Input: part model. Units: mm. Frame: model coordinates. Face numbers are marked on the shaded views. A direction names the side the tool comes from. Round coordinates to 2 decimals unless told otherwise and drop trailing zeros. Loops run counter-clockwise (first coordinate to the right, second up) from the corner with the lowest first, then second, coordinate; pieces in that order, holes last. Notation, with made-up numbers: (76, -35) -> (91, -35) arc R27 cw to (91, -4) -> close; hole circle Ø5 at (-21.5, -36.5). An arc over 180 degrees is marked (long way). Answer in a Markdown table with one row per item. Add a question column.
Q1. Pin query (flat end, axial travel): pin 1 (6 mm diameter, centred on y = -5.5, z = 9.5, fed in from +X); pin 2 (5 mm diameter, centred on x = 10.5, z = 38, fed in from -Y); pin 3 (5 mm diameter, centred on x = 11, z = 13.5, fed in from +Y). Return the tip coordinate at first contact, or that it passes through.
Q2. Section B-B, the plane y = -13.5. Output: boundary loops of the cut face in (x, z), and give its area (3 significant figures).
Q3. Ray query, L1, parallel to Y at x = 20.75, z = 8.5 (3 decimals); L2, parallel to X at y = -14.75, z = 41.5; L3, parallel to Z at x = 18.5, y = -10.5. Return the intervals inside material, ascending. Write a range as from..to.
Q4. Section A-A, the plane z = 11.5. Output: boundary loops of the cut face in (x, y) (3 decimals), and give its area (3 significant figures).
Q5. Reachability of the marked faces 1, 2 and 3 from +Z, -Z, +X, -X, +Y, -Y: full face, straight path, thin tool, end or side. Return the list, or none.
Q6. Mould query, pull axis X, two halves, no side actions, for the marked faces 4, 5, 6 and 7. Classes: pulls with the +X half, pulls with the -X half, needs draft (parallel to the pull), parting line crosses it, or undercut.
Q7. Section C-C, the plane x = 20.25. Output: boundary loops of the cut face in (y, z) (3 decimals).
Q8. Section D-D, the plane z = 7. Output: boundary loops of the cut face in (x, y).
```python
from build123d import *

# Parameters (mm, degrees)
F0_W      = 25.4
F0_H      = 25.4
F1_DEPTH  = 5.08
F2_W      = 20.32
F2_H      = 20.32
F3_DEPTH  = 2.54
F4_W      = 10.16
F4_H      = 10.16
F5_DEPTH  = 10.16
F6_W      = 5.08
F6_H      = 5.08
F7_DEPTH  = 25.4
F8_W      = 2.54
F8_H      = 2.54
F9_DEPTH  = 5.08
F10_R     = 0.635
F11_DEPTH = 0.254
F13_R     = 2.2046300475
F14_DEPTH = 25.4


# Not quite as in the source:
# - a fillet or chamfer that OpenCascade refuses, or shapes differently, is made with other operations: its cross-section is extruded or revolved along the edge and cut away or added


with BuildPart() as f1:
    # F0 (on Top) → F1 (new body)
    with BuildSketch(Plane.XY):
        with Locations((12.7, -12.7)):
            Rectangle(F0_W, F0_H)
    extrude(amount=F1_DEPTH)

    # F2 (on face) → F3 (join)
    with BuildSketch(Plane.XY.offset(5.08)):
        with Locations((12.7, -12.7)):
            Rectangle(F2_W, F2_H)
    extrude(amount=F3_DEPTH)

    # F4 (on face) → F5 (join)
    with BuildSketch(Plane.XY.offset(7.62)):
        with Locations((12.7, -12.7)):
            Rectangle(F4_W, F4_H)
    extrude(amount=F5_DEPTH)

    # F6 (on face) → F7 (join)
    with BuildSketch(Plane.XY.offset(17.78)):
        with Locations((12.7, -12.7)):
            Rectangle(F6_W, F6_H)
    extrude(amount=F7_DEPTH)

    # F8 (on face) → F9 (join)
    with BuildSketch(Plane.XY.offset(7.62)):
        with Locations((4.445, -4.445)):
            Rectangle(F8_W, F8_H)
        with Locations((20.955, -4.445)):
            Rectangle(F8_W, F8_H)
        with Locations((20.955, -20.955)):
            Rectangle(F8_W, F8_H)
        with Locations((4.445, -20.955)):
            Rectangle(F8_W, F8_H)
    extrude(amount=F9_DEPTH)

    # F10 (on face) → F11 (join)
    with BuildSketch(Plane.XZ.offset(22.225)):
        with Locations((4.445, 11.43)):
            Circle(F10_R)
    extrude(amount=F11_DEPTH)

    # F12: fillet of radius 0.8636 on 1 edges, made by hand


with BuildPart() as f12_tool2:
    # F12_s3 → F12_t4 (revolve)
    with BuildSketch(Plane.XY.offset(11.43)):
        with BuildLine():
            ThreePointArc((5.08, -21.6154), (4.9031400964, -22.1390344145), (4.445, -22.4481946926))
            Line((4.445, -22.4481946926), (4.445, -22.479))
            Line((4.445, -22.479), (5.08, -22.479))
            Line((5.08, -22.479), (5.08, -21.6154))
        make_face()
    revolve(axis=Axis((4.445, -22.479, 11.43), (0, -1, 0)))

    split(bisect_by=Plane.XZ.offset(22.225), keep=Keep.TOP)


with BuildPart() as f1_1:
    add(f1.part)

    # F12_t1: cut F12_tool2
    add(f12_tool2.part, mode=Mode.SUBTRACT)

    # F13 (on face) → F14 (cut)
    with BuildSketch(Plane.XZ.offset(22.225)):
        with Locations((4.445, 11.43)):
            Circle(F13_R)
    extrude(amount=F14_DEPTH, mode=Mode.SUBTRACT)


solid = f1_1.part
```
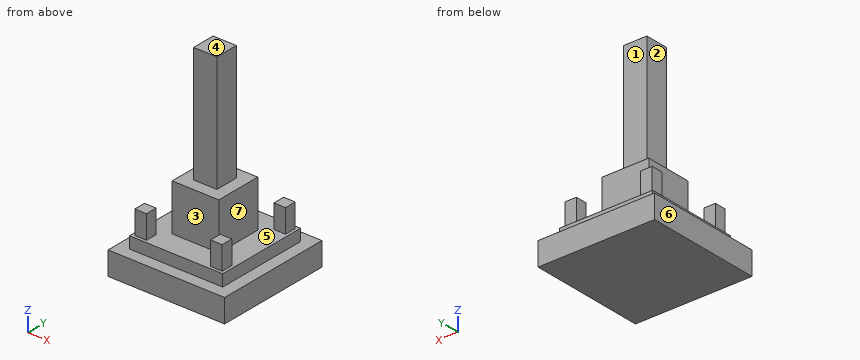
Answer block:
| question | item | result |
|---|---|---|
| 1 | pin 1 | x = 22.86 |
| 1 | pin 2 | y = -15.24 |
| 1 | pin 3 | y = -7.62 |
| 2 | outline | (0, 0) -> (25.4, 0) -> (25.4, 5.08) -> (22.86, 5.08) -> (22.86, 7.62) -> (17.78, 7.62) -> (17.78, 17.78) -> (15.24, 17.78) -> (15.24, 43.18) -> (10.16, 43.18) -> (10.16, 17.78) -> (7.62, 17.78) -> (7.62, 7.62) -> (2.54, 7.62) -> (2.54, 5.08) -> (0, 5.08) -> close |
| 2 | area | 413 mm^2 |
| 3 | L1 | -22.225..-19.685, -5.715..-3.175 |
| 3 | L2 | 10.16..15.24 |
| 3 | L3 | 0..7.62 |
| 4 | outline | (3.175, -22.225) -> (5.715, -22.225) -> (5.715, -19.685) -> (3.175, -19.685) -> close; (3.175, -5.715) -> (5.715, -5.715) -> (5.715, -3.175) -> (3.175, -3.175) -> close; (7.62, -17.78) -> (17.78, -17.78) -> (17.78, -7.62) -> (7.62, -7.62) -> close; (19.685, -22.225) -> (22.225, -22.225) -> (22.225, -19.685) -> (19.685, -19.685) -> close; (19.685, -5.715) -> (22.225, -5.715) -> (22.225, -3.175) -> (19.685, -3.175) -> close |
| 4 | area | 129 mm^2 |
| 5 | face 1 | +Z, +X, -X, +Y |
| 5 | face 2 | +Z, -X, +Y, -Y |
| 5 | face 3 | +Z, +X, -X, -Y |
| 6 | face 4 | needs draft |
| 6 | face 5 | undercut |
| 6 | face 6 | pulls with the -X half |
| 6 | face 7 | pulls with the +X half |
| 7 | outline | (-25.4, 0) -> (0, 0) -> (0, 5.08) -> (-2.54, 5.08) -> (-2.54, 7.62) -> (-3.175, 7.62) -> (-3.175, 12.7) -> (-5.715, 12.7) -> (-5.715, 7.62) -> (-19.685, 7.62) -> (-19.685, 12.7) -> (-22.225, 12.7) -> (-22.225, 7.62) -> (-22.86, 7.62) -> (-22.86, 5.08) -> (-25.4, 5.08) -> close |
| 8 | outline | (2.54, -22.86) -> (22.86, -22.86) -> (22.86, -2.54) -> (2.54, -2.54) -> close |
